```python
from build123d import *

# Parameters (mm, degrees)
SKETCH3_W          = 40
SKETCH3_H          = 1.5
CHAMFER1_SIZE      = 0.45
CUT_EXTRUDE1_DEPTH = 1.19


with BuildPart() as part:
    # Sketch3 → Revolve1 (revolve)
    with BuildSketch(Plane(origin=(0, 0, 0), x_dir=(0, 0, -1), z_dir=(1, 0, 0))):
        with Locations((0, 0.75)):
            Rectangle(SKETCH3_W, SKETCH3_H)
    revolve(axis=Axis((0, 0, -20), (0, 0, 1)))

    # Chamfer1
    chamfer1_edges = [part.edges().sort_by_distance(p)[0] for p in [
        (0, -1.5, -20),
    ]]
    chamfer(chamfer1_edges, length=CHAMFER1_SIZE)

    # Sketch6 → Revolve2 (revolve)
    with BuildSketch(Plane(origin=(0, 0, 0), x_dir=(0, 0, -1), z_dir=(1, 0, 0))):
        Polygon((-20, 3), (-19.8, 3), (-18.3, 1.5), (-18.3, 0), (-20, 0), align=None)
    revolve(axis=Axis((0, 0, -20), (0, 0, 1)))

    # Sketch8 → Cut-Extrude1 (cut)
    with BuildSketch(Plane.XY.offset(20)):
        Polygon((0, 1.154700538), (-1, 0.577350269), (-1, -0.577350269), (0, -1.154700538), (1, -0.577350269), (1, 0.577350269), align=None)
    extrude(amount=-CUT_EXTRUDE1_DEPTH, mode=Mode.SUBTRACT)

    # Cut-Extrude2 cone 1 section (through the dimple's axis) → Cut-Extrude2 (revolve, cut)
    with BuildSketch(Plane(origin=(0, 0, 20), x_dir=(0, -1, 0), z_dir=(1, 0, 0))):
        Polygon((0, 0), (1.154700538, 0), (0, 1.154700538), align=None)
    revolve(axis=Axis((0, 0, 20), (0, 0, -1)), mode=Mode.SUBTRACT)


solid = part.part
```
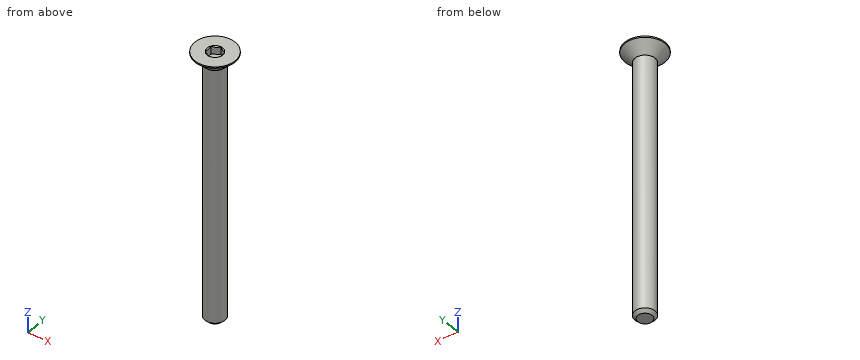
The model under review builds one solid part; all positions refer to its coordinate system, in mm. Round coordinates to 2 decimals unless told otherwise and drop trailing zeros. Loops run counter-clockwise (first coordinate to the right, second up) from the corner with the lowest first, then second, coordinate; pieces in that order, holes last. Notation, with made-up numbers: (-11, 9) -> (40, 9) arc R12 cw to (40, 17) -> close; hole circle Ø6 at (35.5, -18.5). An arc over 180 degrees is marked (long way). Answer as a JSON object with one key per item and string values. Group by question number.
1) For line 1 (Z direction, x = -0.35, y = 0.7); line 2 (Z direction, x = 2.2, y = 0.45); line 3 (Y direction, x = -1.35, z = -18), list the stretches that pass through material, from the lowest coordinate up. Write a range as [from, to].
2) We need section A-A on y = 0. Write out the cut boundary in (x, z), then the cut area to 3 significant figures.
3) We need section B-B on z = 6.5. Write out the cut boundary in (x, y).
4) For pin 1 Ø2 at (x, z) = (0, -6) entering from +Y; pin 2 Ø1 at (y, z) = (1, 3.5) entering from -X; pin 3 Ø3 at (y, z) = (1.5, -7.5) entering from -X, all flat-tipped, find the tip position at first contact; note any pin that passes through.
Result set:
{
 "1": {"line 1": "[-20, 18.81]", "line 2": "[19.05, 20]", "line 3": "[-0.65, 0.65]"},
 "2": {"outline": "(-3, 19.8) -> (-1.5, 18.3) -> (-1.5, -19.55) -> (-1.05, -20) -> (1.05, -20) -> (1.5, -19.55) -> (1.5, 18.3) -> (3, 19.8) -> (3, 20) -> (1.15, 20) -> (1, 19.85) -> (1, 18.81) -> (-1, 18.81) -> (-1, 19.85) -> (-1.15, 20) -> (-3, 20) -> close", "area": "120 mm²"},
 "3": {"outline": "circle Ø3 at (0, 0)"},
 "4": {"pin 1": "y = 1.5", "pin 2": "x = -1.41", "pin 3": "x = -1.5"}
}
